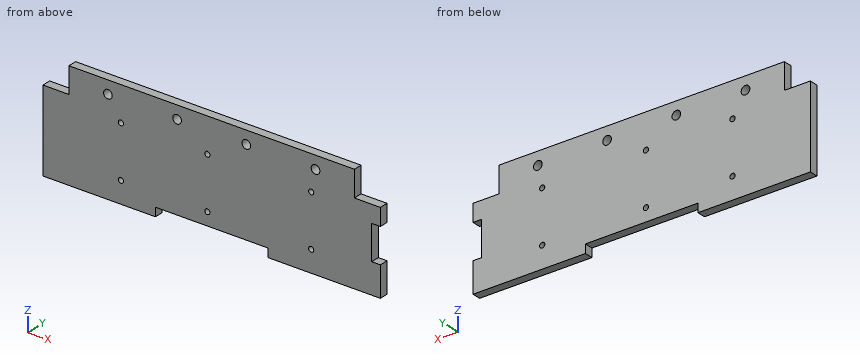
```python
from build123d import *

# Parameters (mm, degrees)
SKETCH1_R           = 5
SKETCH1_R_2         = 3
BOSS_EXTRUDE1_DEPTH = 10
SKETCH2_W           = 30
SKETCH2_H           = 30
CUT_EXTRUDE1_DEPTH  = 10


with BuildPart() as part:
    # Sketch1 → Boss-Extrude1 (new body)
    with BuildSketch(Plane(origin=(0, 0, 0), x_dir=(1, 0, 0), z_dir=(0, 1, 0))):
        Polygon((0, 15), (-390, 15), (-390, 140), (-260, 140), (-260, 130), (-130, 130), (-130, 140), (0, 140), (0, 105), (-10, 105), (-10, 65), (0, 65), align=None)
        with Locations((-315, 30)):
            Circle(SKETCH1_R, mode=Mode.SUBTRACT)
        with Locations((-235, 30)):
            Circle(SKETCH1_R, mode=Mode.SUBTRACT)
        with Locations((-155, 30)):
            Circle(SKETCH1_R, mode=Mode.SUBTRACT)
        with Locations((-75, 30)):
            Circle(SKETCH1_R, mode=Mode.SUBTRACT)
        with Locations((-80, 55)):
            Circle(SKETCH1_R_2, mode=Mode.SUBTRACT)
        with Locations((-200, 55)):
            Circle(SKETCH1_R_2, mode=Mode.SUBTRACT)
        with Locations((-300, 55)):
            Circle(SKETCH1_R_2, mode=Mode.SUBTRACT)
        with Locations((-300, 115)):
            Circle(SKETCH1_R_2, mode=Mode.SUBTRACT)
        with Locations((-200, 115)):
            Circle(SKETCH1_R_2, mode=Mode.SUBTRACT)
        with Locations((-80, 115)):
            Circle(SKETCH1_R_2, mode=Mode.SUBTRACT)
    extrude(amount=BOSS_EXTRUDE1_DEPTH)

    # Sketch2 → Cut-Extrude1 (cut)
    with BuildSketch(Plane.XZ):
        with Locations((-15, -30)):
            Rectangle(SKETCH2_W, SKETCH2_H)
        with Locations((-375, -30)):
            Rectangle(SKETCH2_W, SKETCH2_H)
    extrude(amount=-CUT_EXTRUDE1_DEPTH, mode=Mode.SUBTRACT)


solid = part.part
```
The listing builds one solid part. Answer for the finished solid, in the listing's coordinates (mm). Coordinates: 2 decimals unless noted, no trailing zeros. Write each loop counter-clockwise with the first axis right and the second up, starting at its lowest first coordinate (ties: lowest second). Pieces come first, ordered by that corner, then holes.
Q1. Find the intervals of material crossed by line 1 along X through (y, z) = (4, -55); line 2 along Z through (x, y) = (-75, 3.5); line 3 along Z through (x, y) = (-155, 3.5), in increasing order.
Returned:
line 1: x = -390 to -303, -297 to -203, -197 to -83, -77 to 0
line 2: z = -140 to -35, -25 to -15
line 3: z = -130 to -35, -25 to -15
Q2. Section D-D, the plane z = -78 is taken. Write down the section's boundary in (x, y).
Returned:
outline: (-390, 0) - (-10, 0) - (-10, 10) - (-390, 10) - close
Q3. Section C-C, the plane x = -315 is taken. Write down the section's boundary in (y, z), then the cut area to 3 significant figures.
Returned:
outline: (0, -140) - (10, -140) - (10, -35) - (0, -35) - close; (0, -25) - (10, -25) - (10, -15) - (0, -15) - close
area: 1,150 mm2
Q4. Section B-B, the plane y = 2.75 is taken. Give the number of separate pieces and of enclosed holes in the cut face, then the cut area to 3 significant figures.
Returned:
separate pieces: 1
enclosed holes: 10
area: 44,800 mm2
Q5. Section A-A, the plane x = -235 is taken. Write down the section's boundary in (y, z).
Returned:
outline: (0, -130) - (10, -130) - (10, -35) - (0, -35) - close; (0, -25) - (10, -25) - (10, -15) - (0, -15) - close
Q6. Given P1, Ø5, axis at y = 8.5, z = -28.5, coming from the -X side; P2, Ø5, axis at x = -140, y = 2, coming from the -Z side; P3, Ø5, axis at y = 3, z = -30, coming from the +X side, each flat-ended and moving along its own axis, determine where each tip first touches the part or whether it passes through.
Returned:
P1: stops at x = -360
P2: stops at z = -130
P3: stops at x = -30
